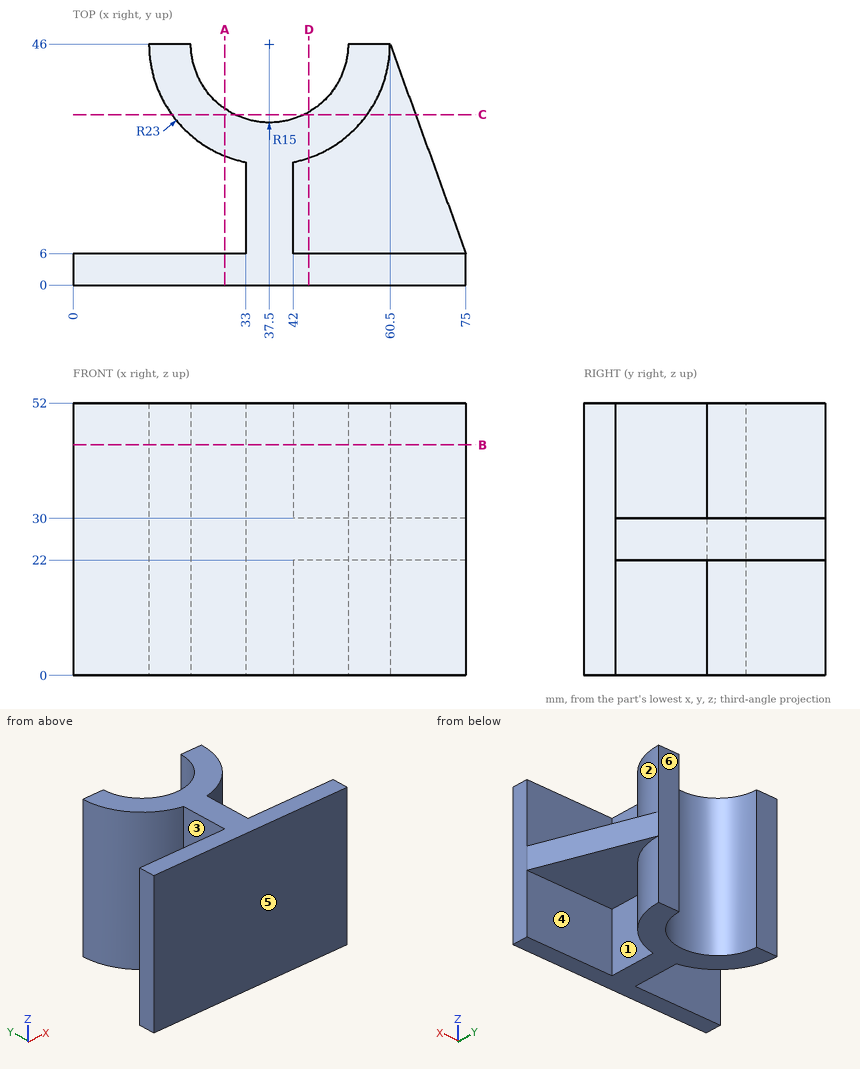
Study the drawing (mm; zero at the part's minimum x, y, z) and answer. A direction names the side the tool comes from. Coordinates: 2 decimals unless noted, no trailing zeros. Order: outer loops, then holes, each group sorted by start corner. A loop starts at its lowest first (then second) coordinate and runs counter-clockwise, first axis right, second up. Notation, with made-up numbers: (79, 9.5) -> (123, 9.5) arc R29 cw to (123, 45.5) -> close; hole circle Ø2 at (79.5, 80.25). An arc over 180 degrees is marked (long way). Answer in a Markdown table with one row per item. Add a question column.
Item 1: Each of these flat-tipped pins is pushed along its axis until it touches: P1, Ø5, axis at y = 38.5, z = 34.5, coming from the -X side; P2, Ø8.5, axis at y = 12, z = 12.5, coming from the +X side; P3, Ø5, axis at y = 13, z = 32.5, coming from the -X side. Where does it stop, or does it pass through?
Item 2: Determine the mould class of the marked faces 4, 5 and 6 for opening direction Y: +Y half, -Y half, draft (parallel to the pull), parting line (faces both ways), or undercut.
Item 3: Find section A-A (x = 29). Write down the section's boundary in (y, z), then the cut area to 3 significant figures.
Item 4: Find section C-C (y = 32.5). Write down the section's boundary in (x, z), then the cut area to 3 significant figures.
Item 5: Which of the six approach directions +Z, -Z, +X, -X, +Y, -Y give full straight-line access (tool end or side, diameter ignored) to the marked faces 1, 2 and 3?
Item 6: Find the intervals of material crossed by L1, parallel to X at y = 7, z = 47.5; L2, parallel to Y at x = 48, z = 33; L3, parallel to Y at x = 63.5, z = 36, in increasing order. Write a range as from..to.
Item 7: Find section D-D (x = 45). Write down the section's boundary in (y, z), then the cut area to 3 significant figures.
Item 8: Find section B-B (z = 44). Write down the section's boundary in (x, y), then the cut area to 3 significant figures.
Result set:
| question | item | result |
|---|---|---|
| 1 | P1 | stops at x = 15.05 |
| 1 | P2 | stops at x = 42 |
| 1 | P3 | stops at x = 33 |
| 2 | face 4 | undercut |
| 2 | face 5 | -Y half |
| 2 | face 6 | +Y half |
| 3 | outline | (0, 0) -> (6, 0) -> (6, 52) -> (0, 52) -> close; (24.63, 0) -> (33.64, 0) -> (33.64, 52) -> (24.63, 52) -> close |
| 3 | area | 781 mm² |
| 4 | outline | (18.88, 0) -> (30.96, 0) -> (30.96, 52) -> (18.88, 52) -> close; (44.04, 0) -> (56.12, 0) -> (56.12, 22) -> (65.39, 22) -> (65.39, 30) -> (56.12, 30) -> (56.12, 52) -> (44.04, 52) -> close |
| 4 | area | 1,330 mm² |
| 5 | face 1 | -Z, +X |
| 5 | face 2 | +Z, +X |
| 5 | face 3 | +Z, -Z, -X |
| 6 | L1 | x = 33..42 |
| 6 | L2 | y = 0..6, 25.54..35.29 |
| 6 | L3 | y = 0..6 |
| 7 | outline | (0, 0) -> (6, 0) -> (6, 22) -> (24.26, 22) -> (24.26, 0) -> (33.01, 0) -> (33.01, 52) -> (24.26, 52) -> (24.26, 30) -> (6, 30) -> (6, 52) -> (0, 52) -> close |
| 7 | area | 913 mm² |
| 8 | outline | (0, 0) -> (75, 0) -> (75, 6) -> (42, 6) -> (42, 23.44) arc R23 ccw to (60.5, 46) -> (52.5, 46) arc R15 cw to (22.5, 46) -> (14.5, 46) arc R23 ccw to (33, 23.44) -> (33, 6) -> (0, 6) -> close |
| 8 | area | 1,080 mm² |
